Source: CAD feature listing. Evaluate the final solid. Frame: model axes, mm. Coordinates: 2 decimals unless noted, no trailing zeros. Loops run counter-clockwise (first coordinate to the right, second up) from the corner with the lowest first, then second, coordinate; pieces in that order, holes last. Notation, with made-up numbers: M 27.5,65 L 34.5,65 A14 cw 34.5,82 Z; hole C 7.5,-3 d1. An arc over 180 degrees is marked long. One line per question, with ' | ' between items. Start each with the question number.
1. Mould query, pull axis X, two halves, no side actions, for faces 1 (the flat face through (-6, 376, 22.225)), 2 (the flat face through (-6, 376, 15.875)). Classes: pulls with the +X half, pulls with the -X half, needs draft (parallel to the pull), parting line crosses it, or undercut.
2. Ray query, probe 1 along Y at (x, z) = (258.5, 13.75) (3 decimals); probe 2 along Y at (x, z) = (-104, 19.5). Return the intervals inside material, ascending.
3. Section query B-B, the plane z = 11.25. Output: boundary loops of the cut face in (x, y) (3 decimals), and give its area (3 significant figures).
4. Section query A-A, the plane y = 155. Output: boundary loops of the cut face in (x, z) (3 decimals).
5. Section query C-C, the plane x = 340.5. State how many separate pieces and enclosed holes the cut face has, and give its area (3 significant figures).
```python
from build123d import *

# Parameters (mm, degrees)
F1_DEPTH  = 19.05
F2_W      = 895.35
F2_H      = 19.05
F5_DEPTH  = 19.05
F6_DEPTH  = 38.1
F3_W      = 895.35
F3_H      = 19.05
F7_DEPTH  = 19.05
F4_W      = 895.35
F4_H      = 19.05
F8_DEPTH  = 127
F10_W     = 895.35
F10_H     = 19.05
F11_DEPTH = 19.05
F12_W     = 895.35
F12_H     = 133.35
F13_DEPTH = 3.175
F13_TAPER = 3


# Not quite as in the source:
# - the program builds the solid bodies; features that only make, move or delete a surface that nothing else refers to are left out


with BuildPart() as f1:
    # F0 (on Top) → F1 (new body)
    with BuildSketch(Plane.XY):
        Polygon((457.2, -457.2), (457.2, 457.2), (186.2517595291, 457.2), (-457.2, 457.2), (-457.2, -457.2), align=None)
        Polygon((-447.675, 447.675), (186.2517595291, 447.675), (447.675, 447.675), (447.675, -447.675), (-447.675, -447.675), align=None, mode=Mode.SUBTRACT)
    extrude(amount=F1_DEPTH)

    # F3 (on face) → F7 (cut)
    with BuildSketch(Plane.XY.offset(19.05)):
        with Locations((0, 298.0556269322)):
            Rectangle(F3_W, F3_H)
    extrude(amount=-F7_DEPTH, mode=Mode.SUBTRACT)

    # F4 (on face) → F8 (cut)
    with BuildSketch(Plane.XY.offset(19.05)):
        with Locations((0, 298.0556269322)):
            Rectangle(F4_W, F4_H)
    extrude(amount=-F8_DEPTH, mode=Mode.SUBTRACT)

    # F10 (on face) → F11 (cut)
    with BuildSketch(Plane.XY.offset(19.05)):
        with Locations((0, 298.0556269322)):
            Rectangle(F10_W, F10_H)
    extrude(amount=-F11_DEPTH, mode=Mode.SUBTRACT)

    # F12 (on face) → F13 (join, symmetric)
    with BuildSketch(Plane.XY.offset(19.05)):
        with Locations((0.6440271378, 375.4221406161)):
            Rectangle(F12_W, F12_H)
    extrude(amount=F13_DEPTH, both=True, taper=F13_TAPER)


with BuildPart() as f5:
    # F2 (on face) → F5 (new body)
    with BuildSketch(Plane.XY.offset(19.05)):
        with Locations((0, 298.0556269322)):
            Rectangle(F2_W, F2_H)
    extrude(amount=F5_DEPTH)

    # F6 (cut): a face of the model
    f6_faces = [f5.faces().sort_by_distance(p)[0] for p in [
        (0, 298.0556269322, 38.1),
    ]]
    extrude(f6_faces, amount=-F6_DEPTH, mode=Mode.SUBTRACT)


solid = f1.part
```
Taken from the geometry:
1) face 1: needs draft | face 2: undercut
2) probe 1: -457.2 to -447.675, 447.675 to 457.2 | probe 2: 308.77 to 442.07
3) outline: M -457.2,-457.2 L 457.2,-457.2 L 457.2,457.2 L -457.2,457.2 Z; hole M -447.675,-447.675 L 447.675,-447.675 L 447.675,447.675 L -447.675,447.675 Z | area: 34,500 mm^2
4) outline: M -457.2,0 L -447.675,0 L -447.675,19.05 L -457.2,19.05 Z; M 447.675,0 L 457.2,0 L 457.2,19.05 L 447.675,19.05 Z
5) separate pieces: 3 | enclosed holes: 0 | area: 1,210 mm^2
